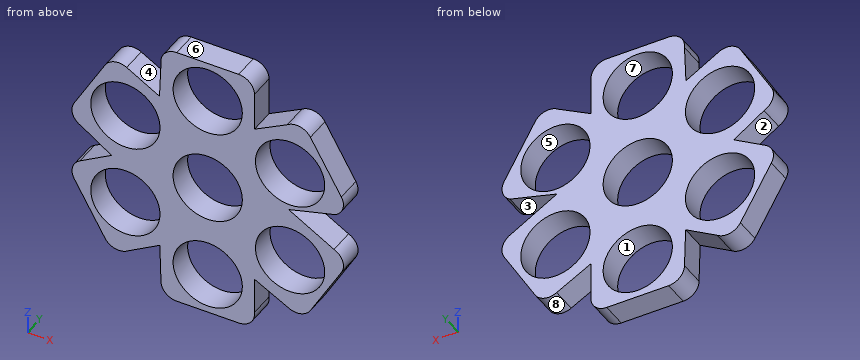
```python
from build123d import *

# Parameters (mm, degrees)
F0_R     = 10.925
F1_DEPTH = 8


# Not quite as in the source:
# - a feature names something its author has since deleted; it is built from what else it names


with BuildPart() as f1:
    # F0 (on Front) → F1 (new body)
    with BuildSketch(Plane.XZ):
        with BuildLine():
            ThreePointArc((-164.4608943756, 109.2849649489), (-165.9253604697, 112.8204988548), (-169.4608943756, 114.2849649489))
            Line((-169.4608943756, 114.2849649489), (-188.9884267566, 114.2849649489))
            ThreePointArc((-188.9884267566, 114.2849649489), (-192.7173858315, 112.6158603567), (-193.95673582, 108.7229106361))
            Line((-193.95673582, 108.7229106361), (-194.4236024673, 97.0532244981))
            Line((-194.4236024673, 97.0532244981), (-204.7831671065, 103.0343219313))
            ThreePointArc((-204.7831671065, 103.0343219313), (-208.577262332, 103.5338240438), (-211.6132941254, 101.2041949124))
            Line((-211.6132941254, 101.2041949123), (-221.3770596376, 84.2928569721))
            ThreePointArc((-221.3770596376, 84.2928569721), (-221.7960530872, 80.2289308569), (-219.0443345156, 77.209146778))
            Line((-219.0443345156, 77.209146778), (-209.5551351868, 70.7485068424))
            Line((-209.5551351868, 70.7485068424), (-219.5310878287, 64.9888878992))
            ThreePointArc((-219.5310878287, 64.9888878992), (-221.8607169602, 61.9528561057), (-221.3612148477, 58.1587608802))
            Line((-221.3612148477, 58.1587608802), (-211.5974493355, 41.24742294))
            ThreePointArc((-211.5974493355, 41.24742294), (-208.2874828054, 38.852600911), (-204.2964137934, 39.7257670587))
            Line((-204.2964137934, 39.7257670587), (-194.3204611514, 45.4853860019))
            Line((-194.3204611514, 45.4853860019), (-193.95673582, 33.1940968847))
            ThreePointArc((-193.95673582, 33.1940968847), (-192.492269726, 29.6585629787), (-188.95673582, 28.1940968847))
            Line((-188.95673582, 28.1940968847), (-169.4292047957, 28.1940968847))
            ThreePointArc((-169.4292047957, 28.1940968847), (-165.7002448161, 29.8632009709), (-164.4608943756, 33.7561511974))
            Line((-164.4608943756, 33.7561511974), (-164.4608943756, 45.2587688032))
            Line((-164.4608943756, 45.2587688032), (-153.6344630891, 39.4447399023))
            ThreePointArc((-153.6344630891, 39.4447399023), (-149.8403678636, 38.9452377897), (-146.8043360702, 41.2748669212))
            Line((-146.8043360702, 41.2748669212), (-137.040570558, 58.1862048614))
            ThreePointArc((-137.040570558, 58.1862048614), (-136.6215771084, 62.2501309766), (-139.37329568, 65.2699150555))
            Line((-139.37329568, 65.2699150555), (-153.7136262629, 73.5493087778))
            Line((-153.7136262629, 73.5493087778), (-138.8865423669, 77.4901739344))
            ThreePointArc((-138.8865423669, 77.4901739344), (-136.5569132354, 80.5262057278), (-137.056415348, 84.3203009533))
            Line((-137.056415348, 84.3203009533), (-146.8201808601, 101.2316388936))
            ThreePointArc((-146.8201808601, 101.2316388936), (-150.1301473902, 103.6264609225), (-154.1212164023, 102.7532947749))
            Line((-154.1212164023, 102.7532947749), (-164.4608943756, 97.2202930303))
            Line((-164.4608943756, 97.2202930303), (-164.4608943756, 109.2849649489))
        make_face()
        with Locations((-179.2088150978, 41.2395309168)):
            Circle(F0_R, mode=Mode.SUBTRACT)
        with Locations((-205.1895772113, 56.2395309168)):
            Circle(F0_R, mode=Mode.SUBTRACT)
        with Locations((-153.2280529843, 56.2395309168)):
            Circle(F0_R, mode=Mode.SUBTRACT)
        with Locations((-205.1895772113, 86.2395309168)):
            Circle(F0_R, mode=Mode.SUBTRACT)
        with Locations((-179.2088150978, 71.2395309168)):
            Circle(F0_R, mode=Mode.SUBTRACT)
        with Locations((-179.2088150978, 101.2395309168)):
            Circle(F0_R, mode=Mode.SUBTRACT)
        with Locations((-153.2280529843, 86.2395309168)):
            Circle(F0_R, mode=Mode.SUBTRACT)
    extrude(amount=F1_DEPTH)


solid = f1.part
```
Verification items for the finished model (mm, model axes). Face numbers are marked on the shaded views. A direction names the side the tool comes from. Round coordinates to 2 decimals unless told otherwise and drop trailing zeros. Order: outer loops, then holes, each group sorted by start corner. A loop starts at its lowest first (then second) coordinate and runs counter-clockwise, first axis right, second up. Notation, with made-up numbers: (75.25, 32) - (91.25, 32) arc R18 ccw to (91.25, 54) - close; hole circle Ø1 at (79, -36). An arc over 180 degrees is marked (long way). Use CSV: the item, a comma, the result in double quotes.
(1) Access from +Z, -Z, +X, -X, +Y, -Y to the whole of each face (thin tool, end or side, straight path). Record for the marked faces 1, 2, 3 and 4.
Entries:
face 1,"+Y, -Y"
face 2,"-X, +Y, -Y"
face 3,"+X, +Y, -Y"
face 4,"+Z, +Y, -Y"
(2) Section check D-D on z = 68.5. Record the boundary of the cut face in (x, y), and give its area (3 significant figures).
Entries:
outline,"(-213.45, -8) - (-189.78, -8) - (-189.78, 0) - (-213.45, 0) - close; (-168.63, -8) - (-144.97, -8) - (-144.97, 0) - (-168.63, 0) - close"
area,"379 mm^2"
(3) Section check C-C on x = -208. Record the boundary of the cut face in (y, z), and give its area (3 significant figures).
Entries:
outline,"(-8, 38.8) - (0, 38.8) - (0, 45.68) - (-8, 45.68) - close; (-8, 66.8) - (0, 66.8) - (0, 75.68) - (-8, 75.68) - close; (-8, 96.8) - (0, 96.8) - (0, 103.65) - (-8, 103.65) - close"
area,"181 mm^2"
(4) Gauge pin test, flat ends, axial feed: pin 1 Ø1.5 at (y, z) = (-4.5, 94) entering from +X; pin 2 Ø1.5 at (x, y) = (-152.5, -1) entering from +Z; pin 3 Ø4 at (y, z) = (-5, 39.5) entering from +X. Record the tip position at first contact, or that the pin passes through.
Entries:
pin 1,"x = -142.21"
pin 2,"z = 103.7"
pin 3,"x = -146.67"
(5) Section check A-A on x = -151. Record the boundary of the cut face in (y, z), and give its area (3 significant figures).
Entries:
outline,"(-8, 38.78) - (0, 38.78) - (0, 45.54) - (-8, 45.54) - close; (-8, 66.93) - (0, 66.93) - (0, 71.98) - (-8, 71.98) - close; (-8, 74.27) - (0, 74.27) - (0, 75.54) - (-8, 75.54) - close; (-8, 96.93) - (0, 96.93) - (0, 103.73) - (-8, 103.73) - close"
area,"159 mm^2"
(6) Mould release check, pull along Z, two halves, no side actions. Record for the marked faces 5, 6, 7 and 8: released by +Z, released by -Z, zero draft, split by the parting line, or undercut.
Entries:
face 5,"undercut"
face 6,"released by +Z"
face 7,"undercut"
face 8,"released by -Z"
(7) Section check B-B on z = 94. Record the boundary of the cut face in (x, y) (3 decimals), and give its area (3 significant figures).
Entries:
outline,"(-215.773, -8) - (-212.879, -8) - (-212.879, 0) - (-215.773, 0) - close; (-197.5, -8) - (-187.391, -8) - (-187.391, 0) - (-197.5, 0) - close; (-171.027, -8) - (-160.918, -8) - (-160.918, 0) - (-171.027, 0) - close; (-145.538, -8) - (-142.645, -8) - (-142.645, 0) - (-145.538, 0) - close"
area,"208 mm^2"
(8) Thickness scan on probe 1 along Z at (x, y) = (-149, -0.5); probe 2 along X at (y, z) = (-6.75, 65); probe 3 along Z at (x, y) = (-158.5, -5.75). Record the ranges inside material, lowest first. Write a range as from..to.
Entries:
probe 1,"39.25..46.17, 66.31..70.83, 74.8..76.17, 96.31..103.25"
probe 2,"-219.51..-211.72, -198.66..-188.18, -170.24..-159.76, -146.7..-138.84"
probe 3,"42.06..46.67, 65.81..76.67, 95.81..100.41"
